Source: three-view drawing plus pictorial views. Frame: mm from the lowest corner of the part. Round coordinates to 2 decimals unless told otherwise and drop trailing zeros. Order: outer loops, then holes, each group sorted by start corner. A loop starts at its lowest first (then second) coordinate and runs counter-clockwise, first axis right, second up. Notation, with made-up numbers: (31, 26.5) - (61, 26.5) arc R16 cw to (61, 52.5) - close; hole circle Ø4 at (46.5, 23). An arc over 180 degrees is marked (long way). Use one line per item in the form item = value. Start each with the question number.
Q1. Cut plane B-B, the plane x = 12.5. Return the cut outline in (y, z), and give its area (3 significant figures).
Q2. Cut plane C-C, the plane z = 41. Return the cut outline in (x, y).
Q3. Pin query (flat end, axial travel): pin 1 Ø1 at (y, z) = (1, 41.5) entering from +X. Return the tip coordinate at first contact, or that it passes through.
Q4. Cut plane A-A, the plane y = 0.5. Return the cut outline in (x, z) (1 decimal).
Q5. Ray query, line 1 (Z direction, x = 39, y = 1.9) (1 decimal); line 2 (X direction, y = 1, z = 34); line 3 (Z direction, x = 43.5, y = 0.4). Return the intervals inside material, ascending. Write a range as [from, to].
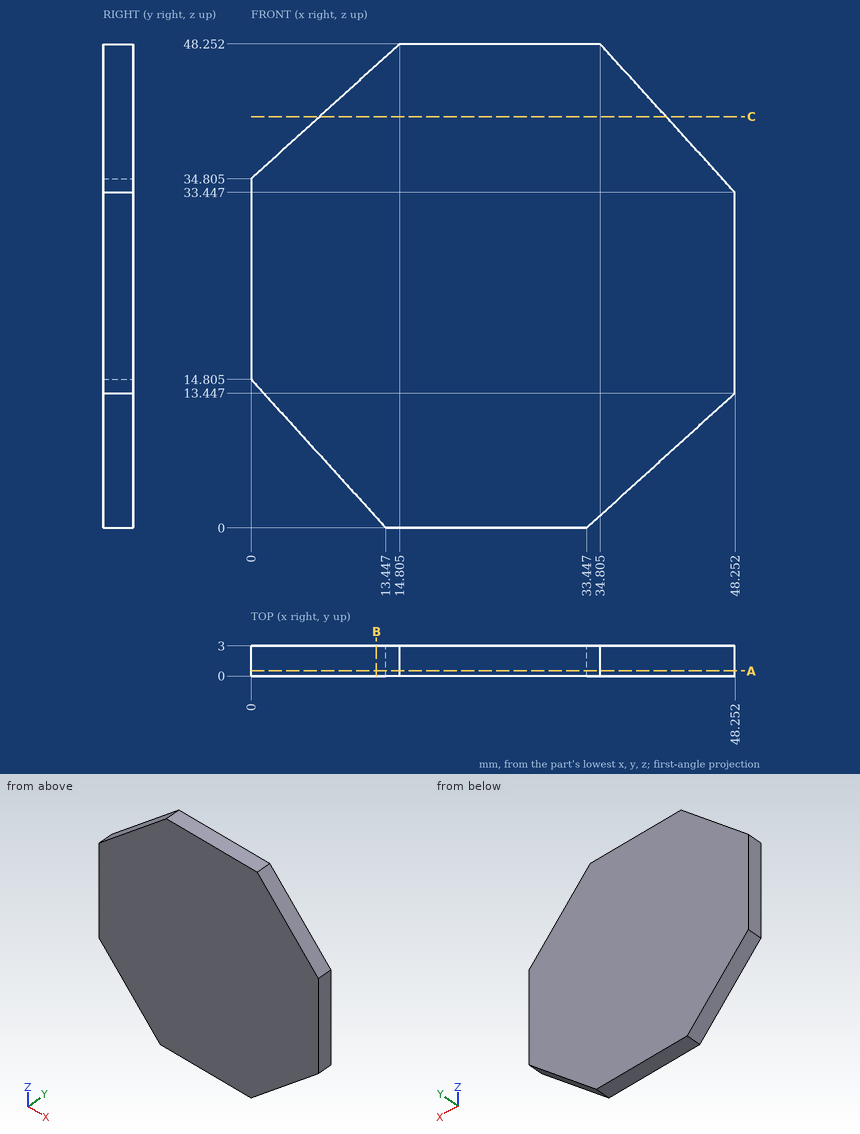
Completed:
q1.outline = (0, 1.04) - (3, 1.04) - (3, 46.16) - (0, 46.16) - close
q1.area = 135 mm2
q2.outline = (6.82, 0) - (41.39, 0) - (41.39, 3) - (6.82, 3) - close
q3.pin_1 = 41.39
q4.outline = (0, 14.8) - (13.4, 0) - (33.4, 0) - (48.3, 13.4) - (48.3, 33.4) - (34.8, 48.3) - (14.8, 48.3) - (0, 34.8) - close
q5.line_1 = [5, 43.6]
q5.line_2 = [0, 47.75]
q5.line_3 = [9.13, 38.68]
